Input: part model. Units: mm. Frame: model coordinates. Face numbers are marked on the shaded views. A direction names the side the tool comes from. Round coordinates to 2 decimals unless told otherwise and drop trailing zeros. Loops run counter-clockwise (first coordinate to the right, second up) from the corner with the lowest first, then second, coordinate; pieces in that order, holes last. Notation, with made-up numbers: (-1.75, 35.5) -> (31.25, 35.5) arc R16 cw to (31.25, 53.5) -> close; hole circle Ø6 at (-35.5, 79). An arc over 180 degrees is marked (long way). Answer as a JSON object with one key per item and string values.
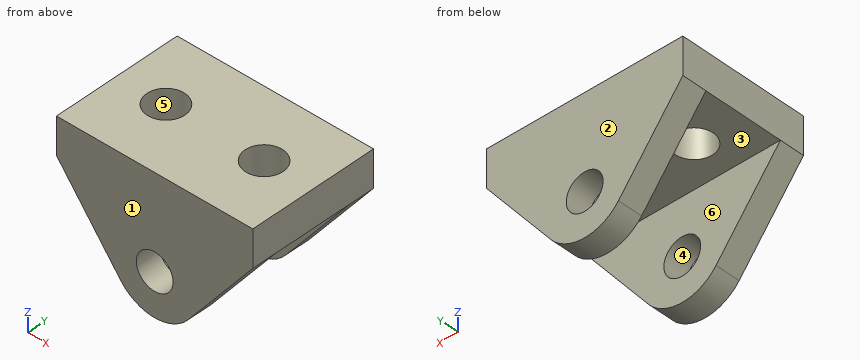
```python
from build123d import *

# Parameters (mm, degrees)
SKETCH1_R           = 4.7625
BOSS_EXTRUDE1_DEPTH = 33.528
CUT_EXTRUDE1_DEPTH  = 71.206566048
SKETCH3_R           = 4.9022
CUT_EXTRUDE2_DEPTH  = 9.4996


with BuildPart() as part:
    # Sketch1 → Boss-Extrude1 (new body)
    with BuildSketch(Plane(origin=(0, 0, 0), x_dir=(1, 0, 0), z_dir=(0, 1, 0))):
        with BuildLine():
            Line((0, 0), (50.8, 0))
            Line((50.8, 0), (50.8, 9.4996))
            Line((50.8, 9.4996), (34.143571574, 30.734397216))
            ThreePointArc((34.143571574, 30.734397216), (25.4, 34.9885), (16.656428426, 30.734397216))
            Line((16.656428426, 30.734397216), (0, 9.4996))
            Line((0, 9.4996), (0, 0))
        make_face()
        with Locations(Location((25.4, 23.876, 0), (0, 0, 270))):
            Circle(SKETCH1_R, mode=Mode.SUBTRACT)
    extrude(amount=BOSS_EXTRUDE1_DEPTH)

    # Sketch2 → Cut-Extrude1 (cut, through all)
    with BuildSketch(Plane(origin=(50.8, 0, 0), x_dir=(0, 0, -1), z_dir=(1, 0, 0))):
        Polygon((9.4996, 16.764), (9.4996, 27.1145), (34.9885, 27.1145), (34.9885, 6.4135), (9.4996, 6.4135), align=None)
    extrude(amount=-CUT_EXTRUDE1_DEPTH, mode=Mode.SUBTRACT)

    # Sketch3 → Cut-Extrude2 (cut)
    with BuildSketch(Plane(origin=(0, 0, -9.4996), x_dir=(-1, 0, 0), z_dir=(0, 0, -1))):
        with Locations((-38.1, 16.764)):
            Circle(SKETCH3_R)
        with Locations((-12.7, 16.764)):
            Circle(SKETCH3_R)
    extrude(amount=-CUT_EXTRUDE2_DEPTH, mode=Mode.SUBTRACT)


solid = part.part
```
1) Draft query along Y for the marked faces 1, 2, 3 and 4. Return one class per face: +Y half, -Y half, draft (parallel to the pull), parting line (faces both ways), or undercut.
Output:
{"face 1": "-Y half", "face 2": "+Y half", "face 3": "undercut", "face 4": "draft"}
2) Section B-B, the plane x = 38.1. Output: boundary loops of the cut face in (y, z).
Output:
{"outline": "(0, -25.69) -> (6.41, -25.69) -> (6.41, -9.5) -> (11.86, -9.5) -> (11.86, 0) -> (0, 0) -> close; (21.67, -9.5) -> (27.11, -9.5) -> (27.11, -25.69) -> (33.53, -25.69) -> (33.53, 0) -> (21.67, 0) -> close"}
3) Reachability of the marked faces 5 and 6 from +Z, -Z, +X, -X, +Y, -Y: full face, straight path, thin tool, end or side. Return the list, or none.
Output:
{"face 5": "+Z, -Z", "face 6": "-Z, +X, -X"}
4) Section C-C, the plane z = -22.5. Output: boundary loops of the cut face in (x, y), plus the area to 3 significant figures.
Output:
{"outline": "(10.2, 0) -> (20.84, 0) -> (20.84, 6.41) -> (10.2, 6.41) -> close; (10.2, 27.11) -> (20.84, 27.11) -> (20.84, 33.53) -> (10.2, 33.53) -> close; (29.96, 0) -> (40.6, 0) -> (40.6, 6.41) -> (29.96, 6.41) -> close; (29.96, 27.11) -> (40.6, 27.11) -> (40.6, 33.53) -> (29.96, 33.53) -> close", "area": "273 mm^2"}
5) Ray query, probe 1 along Y at (x, z) = (25, -15); probe 2 along Y at (x, z) = (38, -3); probe 3 along Z at (x, y) = (42.5, 12). Return the intervals inside material, ascending.
Output:
{"probe 1": "y = 0 to 6.41, 27.11 to 33.53", "probe 2": "y = 0 to 11.86, 21.67 to 33.53", "probe 3": "z = -9.5 to 0"}
6) Section D-D, the plane y = 4. Output: boundary loops of the cut face in (x, z) (1 decimal).
Output:
{"outline": "(0, -9.5) -> (16.7, -30.7) arc R11.1 ccw to (34.1, -30.7) -> (50.8, -9.5) -> (50.8, 0) -> (0, 0) -> close; hole circle Ø9.5 at (25.4, -23.9)"}
7) Contact query for flat-ended pins moving along their axis: P1, Ø11.5, axis at x = 38.1, y = 16.764, coming from the -Z side; P2, Ø3, axis at x = 7.5, y = 7, coming from the -Z side; P3, Ø1.5, axis at x = 20.5, y = 29.5, coming from the -Z side. Output: stop coordinate, or through.
Output:
{"P1": "stops at z = -9.5", "P2": "stops at z = -20.82", "P3": "stops at z = -34.18"}
8) Section A-A, the plane x = 25.4. Output: boundary loops of the cut face in (y, z).
Output:
{"outline": "(0, -34.99) -> (6.41, -34.99) -> (6.41, -28.64) -> (0, -28.64) -> close; (0, -19.11) -> (6.41, -19.11) -> (6.41, -9.5) -> (27.11, -9.5) -> (27.11, -19.11) -> (33.53, -19.11) -> (33.53, 0) -> (0, 0) -> close; (27.11, -34.99) -> (33.53, -34.99) -> (33.53, -28.64) -> (27.11, -28.64) -> close"}
